Autodesk Inventor part; units mm, degrees
ref_plane "Work Plane1" through (0, 0, 0) normal (0, 0.5, 0.866) x (1, 0, 0)
ref_plane "YZ Plane" through (0, 0, 0) normal (1, 0, 0) x (0, 1, 0)
ref_plane "XZ Plane" through (0, 0, 0) normal (0, 1, 0) x (-1, 0, 0)
sketch "Sketch1" plane through (0, 0, 0) normal (0, 0, 1) x (1, 0, 0)
  line L0 (-3.0696, 0) -> (40, 0)
  line L1 (40, 0) -> (40, 4)
  line L2 (40, 4) -> (12, 4)
  line L3 (12, 4) -> (11.2332, 4)
  line L4 (11.2332, 4) -> (0.4, 4)
  line L5 (0, 4.4) -> (0, 6.5)
  line L6 (0, 6.5) -> (-8, 6.5)
  line L7 (-8, 6.5) -> (-8, 3.3435)
  line L8 (-8, 3.3435) -> (-5, 3.3435)
  line L9 (-5, 3.3435) -> (-3.0696, 0)
  line L10 (-17.6, 0) -> (49.6, 0)
  line L11 (0, -1.3) -> (0, 7.8)
  line L12 (12, 4) -> (0, 4) construction
  arc A0 (0, 4.4) -> (0.4, 4) centre (0.4, 4.4) ccw
  point P0 (0, 4)
  dimension "d1" = 28
  dimension "d2" = 0.7668
  dimension "d3" = 8
  dimension "d4" = 3
  dimension "d5" = 60
  dimension "d6" = 8
  dimension "d7" = 8
  dimension "d8" = 6.687
  dimension "d9" = 13
  dimension "d20" = 40
  dimension "d34" = 0.4
revolve "Body" add sketch "Sketch1" angle 360 about axis through (-3.0696, 0, 0) along (1, 0, 0)
sketch "Sketch2" plane through (-8, 0, 0) normal (-1, 0, 0) x (0, 0, 1)
  line L0 (0, -9.1) -> (0, 9.1)
  line L1 (-9.1, 0) -> (9.1, 0)
  circle A0 centre (0, 0) radius 3.3435
  circle A1 centre (0, 0) radius 2.39
  line L2 (0, 0) -> (5.8463, 3.3754) construction
  line L3 (0, 0) -> (2.9613, 5.1292) construction
  arc A2 (1.9271, 2.2791) -> (1.0103, 2.8085) centre (1.3978, 2.421) ccw
  arc A3 (2.9373, -0.5293) -> (2.9373, 0.5293) centre (2.7955, 0) ccw
  arc A4 (1.9271, 2.2791) -> (2.9373, 0.5293) centre (3.3071, 1.9094) ccw
  arc A5 (-1.0103, 2.8085) -> (-1.9271, 2.2791) centre (-1.3978, 2.421) ccw
  arc A6 (-2.9373, 0.5293) -> (-2.9373, -0.5293) centre (-2.7955, 0) ccw
  arc A7 (-2.9373, 0.5293) -> (-1.9271, 2.2791) centre (-3.3071, 1.9094) ccw
  arc A8 (-1.9271, -2.2791) -> (-1.0103, -2.8085) centre (-1.3978, -2.421) ccw
  arc A9 (-1.9271, -2.2791) -> (-2.9373, -0.5293) centre (-3.3071, -1.9094) ccw
  arc A10 (-2.9373, 0.5293) -> (-2.9373, -0.5293) centre (-2.7955, 0) ccw
  arc A11 (1.0103, -2.8085) -> (1.9271, -2.2791) centre (1.3978, -2.421) ccw
  arc A12 (2.9373, -0.5293) -> (2.9373, 0.5293) centre (2.7955, 0) ccw
  arc A13 (2.9373, -0.5293) -> (1.9271, -2.2791) centre (3.3071, -1.9094) ccw
  arc A14 (-1.0103, 2.8085) -> (1.0103, 2.8085) centre (0, 3.8187) ccw
  arc A15 (1.0103, -2.8085) -> (-1.0103, -2.8085) centre (0, -3.8187) ccw
  dimension "d35" = 4.78
  dimension "d36" = 30
  dimension "d37" = 60
  dimension "d38" = 0.548
extrude "Slot" add sketch "Sketch2" against normal up to next contours A0 A8 A15 L0 | L0 A15 A11 A0 | A0 A6 A9 A8 | A11 A13 A3 A0 | A0 A5 A7 A6 | A3 A4 A2 A0 | A14 A5 A0 L0 | L0 A0 A2 A14
fillet "Fillet1" radius 0.5 1 edges at (-8, -6.5, 0)
thread "Thread"
chamfer "Chamfer1" distance 0.7668 distance2 0.7669 1 edges at (40, -4, 0) measured on face at (40, -0.998, -0.8842)
ref_plane "Work Plane1" through (0, 0, 0) normal (0, 0.5, 0.866) x (1, 0, 0)
equation "\"d1\" = GEL"
equation "\"d2\" = GAL"
equation "\"d3\" = KOH"
equation "\"d4\" = INTI"
equation "\"d6\" = GD"
equation "\"d7\" = BDM"
equation "\"d8\" = E0"
equation "\"d9\" = KOD"
equation "\"d20\" = NLG"
equation "\"d34\" = R"
equation "\"d35\" = SW"
equation "\"d38\" = RRK"
equation "\"d17\" = RR"
equation "\"d13\" = GEL"
equation "\"d15\" = -0.5 * SPD + 0.5 * GD"
equation "\"GD\" = NND"
equation "\"NLG\" = 40"
equation "\"GEL\" = 28"
equation "\"KOD\" = 13"
equation "\"KOH\" = 8"
equation "\"INTI\" = 3"
equation "\"GAL\" = 0.61345 * PTC"
equation "\"GUL\" = 0.61345 * PTC"
equation "\"BDM\" = NND"
equation "\"SW\" = 4.78"
equation "\"RR\" = 0.5"
equation "\"SPD\" = NND - 1.2269 * PTC"
equation "\"R\" = 0.4"
equation "\"E0\" = 6.687"
equation "\"RRK\" = 0.548"
equation "\"TOA\" = 30deg"
equation "\"GD1\" = THREADDIA - 1.2269 * PTC"
equation "\"THREADDIA\" = 8"
equation "\"FAWI\" = 45deg"
equation "\"ANG\" = 120deg"
equation "\"PTC\" = 1.25"
equation "\"NND\" = 8"
equation "\"KEWI\" = 5deg"
properties part number "Screw GB/T 2171.2 M8 x 40" material "Acciaio, Dolce"
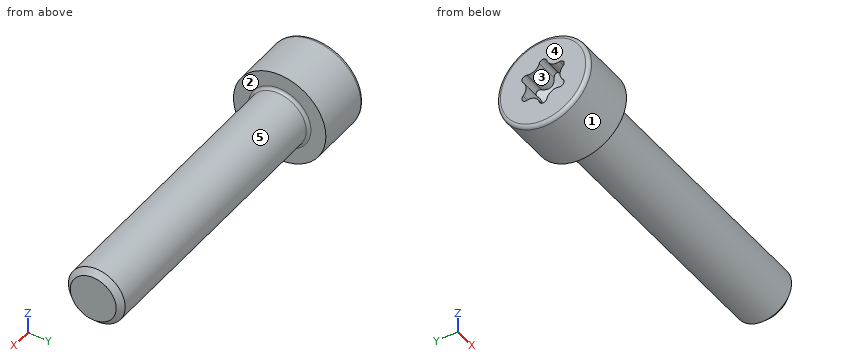
The model under review builds one solid part; all positions refer to its coordinate system, in mm. Face numbers are marked on the shaded views. A direction names the side the tool comes from. Give positions to 0.01 mm unless a question says otherwise; leave off trailing zeros. Write each loop counter-clockwise with the first axis right and the second up, starting at its lowest first coordinate (ties: lowest second). Pieces come first, ordered by that corner, then holes. Notation, with made-up numbers: (70, -4) - (126, -4) arc R31 cw to (126, 28) - close; hole circle Ø5 at (66, 38). An arc over 180 degrees is marked (long way). Answer in a Markdown table with one row per item. Add a question column.
1. Insertion check: P1, Ø3, axis at x = 3.5, y = 3.5, coming from the +Z side; P2, Ø5, axis at x = 11.5, y = -3.5, coming from the +Z side; P3, Ø3, axis at x = 17, z = -1.5, coming from the +Y side; P4, Ø4, axis at y = -4, z = -0.5, coming from the +X side. Each pin has a flat end and moves straight along its axis. Give the tip position at first contact, or say it passes through.
2. We need section A-A on x = 7. Write out the cut boundary in (y, z), then the cut area to 3 significant figures.
3. Tool access review of the marked faces 1 and 2: name each direction out of +Z, -Z, +X, -X, +Y, -Y from which nothing blocks a thin tool from reaching the whole face with its end or side.
4. Draft analysis for pull direction Y (two halves, no side actions). For the marked faces 3, 4 and 5, state which applies: +Y half, -Y half, draft (parallel to the pull), parting line (faces both ways), or undercut.
5. Wall thickness on line 1 along X through (y, z) = (4.5, 3.5); line 2 along Z through (x, y) = (6.5, 0); line 3 along Y through (x, z) = (17, -0.75): over which ranges is each line inside the solid? List them lowest first. Write a range as [from, to].
Ans:
| question | item | result |
|---|---|---|
| 1 | P1 | stops at z = 3.46 |
| 1 | P2 | stops at z = 3.87 |
| 1 | P3 | stops at y = 4 |
| 1 | P4 | stops at x = 40 |
| 2 | outline | circle Ø8 at (0, 0) |
| 2 | area | 50.3 mm^2 |
| 3 | face 1 | +X, -X |
| 3 | face 2 | +X |
| 4 | face 3 | undercut |
| 4 | face 4 | draft |
| 4 | face 5 | parting line |
| 5 | line 1 | x = [-8, 0] |
| 5 | line 2 | z = [-4, 4] |
| 5 | line 3 | y = [-3.93, 3.93] |
